from build123d import *

# Parameters (mm, degrees)
BOSS_EXTRUDE1_DEPTH      = 6.5
BOSS_EXTRUDE1_DEPTH_BACK = 6.5
SKETCH3_R                = 6.5
BOSS_EXTRUDE2_DEPTH      = 4
SKETCH4_R                = 2.5
SKETCH4_R_2              = 1.25
BOSS_EXTRUDE3_DEPTH      = 3
CUT_EXTRUDE1_DEPTH       = 29.901773302
CUT_EXTRUDE1_DEPTH_BACK  = 29.901773302


with BuildPart() as part:
    # Sketch1 → Boss-Extrude1 (new, two sides: drawn at the far end of the back side and taken through both)
    with BuildSketch(Plane.XY.offset(-BOSS_EXTRUDE1_DEPTH_BACK)):
        Polygon((-11.25, -8.5), (11.25, -8.5), (11.25, 8.5), (16.25, 8.5), (16.25, 11), (11.25, 11), (11.25, 16), (-11.25, 16), (-11.25, 11), (-16.25, 11), (-16.25, 8.5), (-11.25, 8.5), align=None)
    extrude(amount=BOSS_EXTRUDE1_DEPTH + BOSS_EXTRUDE1_DEPTH_BACK)

    # Sketch3 → Boss-Extrude2 (add)
    with BuildSketch(Plane(origin=(0, 16, 0), x_dir=(1, 0, 0), z_dir=(0, 1, 0))):
        with Locations((-4.75, 0)):
            Circle(SKETCH3_R)
        with BuildLine():
            Line((-4.75, 3), (2.75, 3))
            ThreePointArc((2.75, 3), (5.75, 0), (2.75, -3))
            Line((2.75, -3), (-4.75, -3))
            ThreePointArc((-4.75, -3), (-7.75, 0), (-4.75, 3))
        make_face()
    extrude(amount=BOSS_EXTRUDE2_DEPTH)

    # Sketch4 → Boss-Extrude3 (add)
    with BuildSketch(Plane(origin=(0, 20, 0), x_dir=(1, 0, 0), z_dir=(0, 1, 0))):
        with Locations(Location((-4.75, 0, 0), (0, 0, 180))):
            Circle(SKETCH4_R)
        with Locations(Location((-4.75, 0, 0), (0, 0, 180))):
            Circle(SKETCH4_R_2, mode=Mode.SUBTRACT)
    extrude(amount=BOSS_EXTRUDE3_DEPTH)

    # Sketch5 → Cut-Extrude1 (cut, two sides: drawn at the far end of the back side and taken through both)
    with BuildSketch(Plane(origin=(0, 0, 0), x_dir=(1, 0, 0), z_dir=(0, 1, 0)).offset(-CUT_EXTRUDE1_DEPTH_BACK)):
        with BuildLine():
            Line((-16.25, 0.5), (-15.45, 0.5))
            ThreePointArc((-15.45, 0.5), (-12.535786438, 0), (-15.45, -0.5))
            Line((-15.45, -0.5), (-16.25, -0.5))
            Line((-16.25, -0.5), (-16.25, 0.5))
        make_face()
        with BuildLine():
            Line((16.25, -0.5), (15.45, -0.5))
            ThreePointArc((15.45, -0.5), (12.535786438, 0), (15.45, 0.5))
            Line((15.45, 0.5), (16.25, 0.5))
            Line((16.25, 0.5), (16.25, -0.5))
        make_face()
    extrude(amount=CUT_EXTRUDE1_DEPTH + CUT_EXTRUDE1_DEPTH_BACK, mode=Mode.SUBTRACT)


solid = part.part
Input: part model. Units: mm. Frame: model coordinates. A direction names the side the tool comes from. Round coordinates to 2 decimals unless told otherwise and drop trailing zeros. Order: outer loops, then holes, each group sorted by start corner. A loop starts at its lowest first (then second) coordinate and runs counter-clockwise, first axis right, second up. Notation, with made-up numbers: (57.5, 83.25) - (97.5, 83.25) arc R9 ccw to (97.5, 100.25) - close; hole circle Ø11 at (-1.75, 54). An arc over 180 degrees is marked (long way). Answer as a JSON object with one key per item and string values. Group by question number.
(1) Cut plane D-D (z = -5.25). Return loops of the section in (x, y), then the cut area to 3 significant figures.
(2) Pin query (flat end, axial travel): P1, Ø2.5, axis at x = -13, z = 0.5, coming from the +Y side; P2, Ø1.9, axis at x = 1.5, y = 17.5, coming from the -Z side; P3, Ø6, axis at x = 7, y = 17.5, coming from the -Z side; P4, Ø6, axis at y = -3, z = 1.5, coming from the -X side. Return the tip coordinate at first contact, or that it passes through.
(3) Reachability of faces 1 (the face through (5.75, 17.97, -0.07)), 2 (the face through (-14, 11, -2)), 3 (the face through (-3.5, 21.48, 0.05)) from +Z, -Z, +X, -X, +Y, -Y: full face, straight path, thin tool, end or side. Return the list, or none.
(4) Cut plane C-C (y = 15). Return loops of the section in (x, z), then the cut area to 4 significant figures.
(5) Cut plane B-B (z = 5.75). Return loops of the section in (x, y), then the cut area to 4 significant figures.
(6) Cut plane A-A (x = -14). Return loops of the section in (y, z).
(7) Draft query along Z for faces 4 (the face through (0, 4, -6.5)), 5 (the face through (-5, 20, 0)), 6 (the face through (11.25, 13, 0)). Return one class per face: released by +Z, released by -Z, zero draft, split by the parting line, or undercut.
(8) Material intervals for probe 1 along Y at (x, z) = (3, -3.75); probe 2 along Y at (x, z) = (-8.5, -1.5); probe 3 along X at (y, z) = (9.2, 0), sorted ascending. Write a range as from..to.
Here are the results:
{
 "1": {"outline": "(-16.25, 8.5) - (-11.25, 8.5) - (-11.25, -8.5) - (11.25, -8.5) - (11.25, 8.5) - (16.25, 8.5) - (16.25, 11) - (11.25, 11) - (11.25, 16) - (-0.92, 16) - (-0.92, 20) - (-8.58, 20) - (-8.58, 16) - (-11.25, 16) - (-11.25, 11) - (-16.25, 11) - close", "area": "607 mm^2"},
 "2": {"P1": "stops at y = 11", "P2": "stops at z = -3.76", "P3": "stops at z = -6.5", "P4": "stops at x = -11.25"},
 "3": {"face 1": "+X, +Y", "face 2": "+Z, -Z, -X, +Y", "face 3": "+Y"},
 "4": {"outline": "(-11.25, -6.5) - (11.25, -6.5) - (11.25, 6.5) - (-11.25, 6.5) - close", "area": "292.5 mm^2"},
 "5": {"outline": "(-16.25, 8.5) - (-11.25, 8.5) - (-11.25, -8.5) - (11.25, -8.5) - (11.25, 8.5) - (16.25, 8.5) - (16.25, 11) - (11.25, 11) - (11.25, 16) - (-1.72, 16) - (-1.72, 20) - (-7.78, 20) - (-7.78, 16) - (-11.25, 16) - (-11.25, 11) - (-16.25, 11) - close", "area": "600.5 mm^2"},
 "6": {"outline": "(8.5, -6.5) - (11, -6.5) - (11, -1.5) - (8.5, -1.5) - close; (8.5, 1.5) - (11, 1.5) - (11, 6.5) - (8.5, 6.5) - close"},
 "7": {"face 4": "released by -Z", "face 5": "undercut", "face 6": "zero draft"},
 "8": {"probe 1": "y = -8.5..16", "probe 2": "y = -8.5..20", "probe 3": "x = -12.54..12.54"}
}
